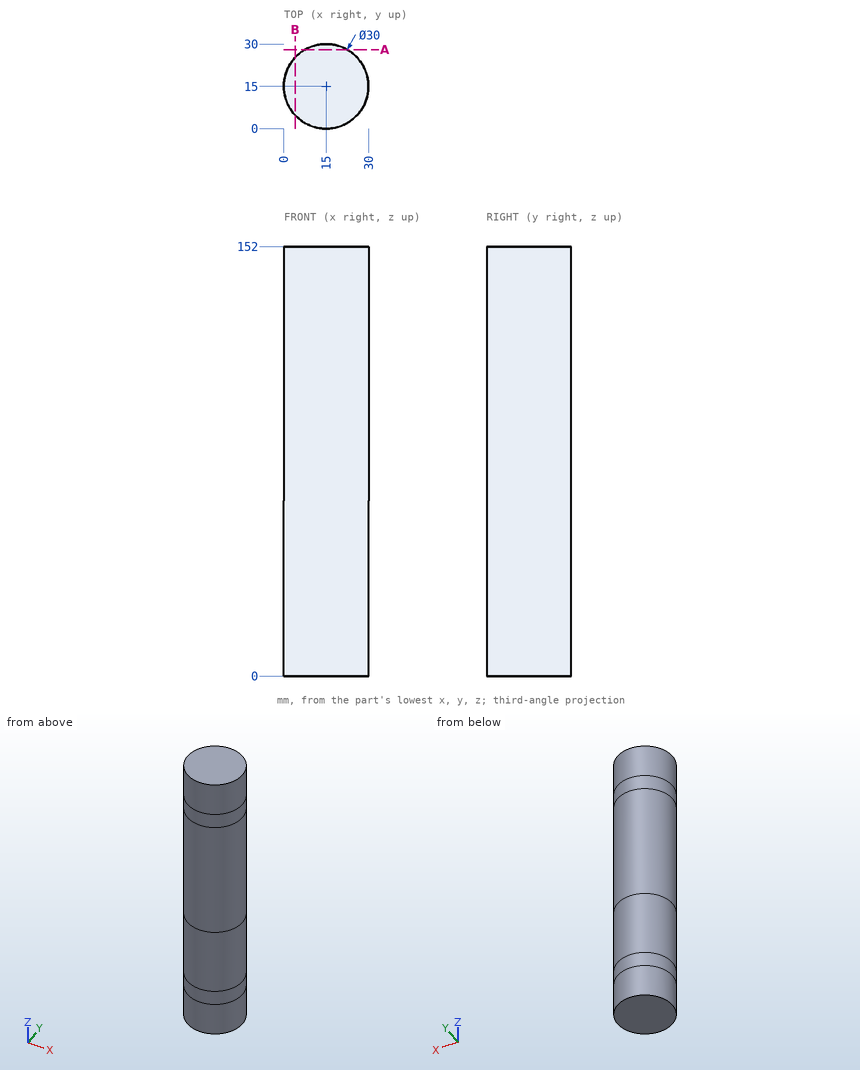
Could you check a few things on this drawing? It's one solid part, dimensions in mm from its lowest x, y, z. Coordinates: 2 decimals unless noted, no trailing zeros. Write each loop counter-clockwise with the first axis right and the second up, starting at its lowest first coordinate (ties: lowest second). Pieces come first, ordered by that corner, then holes.
1) If I drill on line 1 (Y direction, x = 15.25, z = 37.5); line 2 (X direction, y = 15.5, z = 30); line 3 (Y direction, x = 23.75, z = 128), over which ranges is the centre line in solid material (lowest first)?
Filled in:
line 1: y = 0 to 30
line 2: x = 0.01 to 29.99
line 3: y = 2.82 to 27.18
2) If we section it at A-A (y = 28): List the corners of the cut face in (x, z) for me.
Filled in:
outline: (7.52, 0) - (22.48, 0) - (22.48, 152) - (7.52, 152) - close
3) I'm going to push flat-ended pins straight in: pin 1 (6 mm diameter, centred on x = 11.5, z = 32, fed in from -Y); pin 2 (10 mm diameter, centred on x = 20.5, z = 37.5, fed in from +Y); pin 3 (1 mm diameter, centred on y = 26, z = 52.5, fed in from -X). Where does each tip first touch, or does it pass through?
Filled in:
pin 1: stops at y = 0.01
pin 2: stops at y = 29.99
pin 3: stops at x = 4.29
4) If we section it at B-B (x = 4): List the corners of the cut face in (y, z) for me.
Filled in:
outline: (4.8, 0) - (25.2, 0) - (25.2, 152) - (4.8, 152) - close
